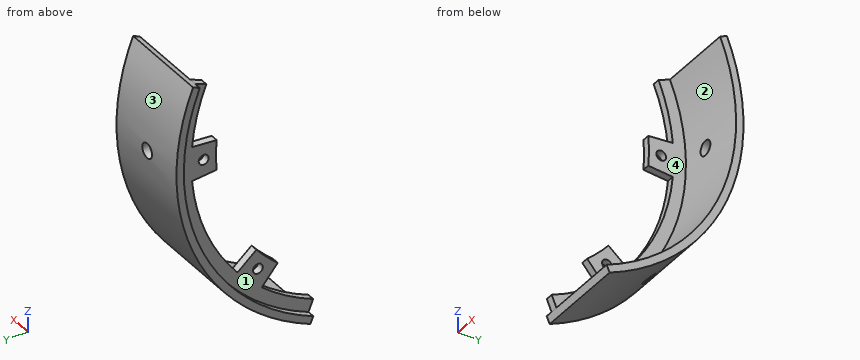
```python
from build123d import *

# Parameters (mm, degrees)
SKETCH5_R                = 2
BOSS_EXTRUDE2_DEPTH      = 3
BOSS_EXTRUDE3_DEPTH      = 30.8
BOSS_EXTRUDE3_DEPTH_BACK = 6
CUT_EXTRUDE1_START       = 84.947042212
CUT_EXTRUDE1_DEPTH       = 3.052957992
CIRPATTERN1_COUNT        = 8


# Read off the part's stored shape, not the designer's step: Cut-Extrude1
with BuildPart() as part:
    # Sketch5 → Boss-Extrude2 (new body)
    with BuildSketch(Plane(origin=(0, 0, 0), x_dir=(0, 0, -1), z_dir=(1, 0, 0))):
        with BuildLine():
            Line((-32.528091751, 78.529760263), (-30.614674589, 73.910362601))
            ThreePointArc((-30.614674589, 73.910362601), (-19.014871386, 77.707365585), (-6.97245942, 79.695575847))
            Line((-6.97245942, 79.695575847), (-6.100901992, 69.733628866))
            ThreePointArc((-6.100901992, 69.733628866), (0, 70), (6.100901992, 69.733628866))
            Line((6.100901992, 69.733628866), (6.97245942, 79.695575847))
            ThreePointArc((6.97245942, 79.695575847), (30.614674589, 73.910362601), (51.423008775, 61.28355545))
            Line((51.423008775, 61.28355545), (44.995132678, 53.623111018))
            ThreePointArc((44.995132678, 53.623111018), (49.497474683, 49.497474683), (53.623111018, 44.995132678))
            Line((53.623111018, 44.995132678), (61.28355545, 51.423008775))
            ThreePointArc((61.28355545, 51.423008775), (68.392949654, 41.501860653), (73.910362601, 30.614674589))
            Line((73.910362601, 30.614674589), (78.529760263, 32.528091751))
            ThreePointArc((78.529760263, 32.528091751), (32.528091751, 78.529760263), (-32.528091751, 78.529760263))
        make_face()
        with Locations((0, 75)):
            Circle(SKETCH5_R, mode=Mode.SUBTRACT)
        with Locations((53.033008589, 53.033008589)):
            Circle(SKETCH5_R, mode=Mode.SUBTRACT)
    extrude(amount=BOSS_EXTRUDE2_DEPTH)

    # Sketch6 → Boss-Extrude3 (add, two sides: drawn at the far end of the back side and taken through both)
    with BuildSketch(Plane(origin=(3, 0, 0), x_dir=(0, 0, -1), z_dir=(1, 0, 0)).offset(-BOSS_EXTRUDE3_DEPTH_BACK)):
        with BuildLine():
            Line((-33.776344001, 81.259821474), (-32.528091751, 78.529760263))
            ThreePointArc((-32.528091751, 78.529760263), (32.528091751, 78.529760263), (78.529760263, 32.528091751))
            Line((78.529760263, 32.528091751), (81.259821474, 33.776344001))
            ThreePointArc((81.259821474, 33.776344001), (33.575888915, 81.342852689), (-33.776344001, 81.259821474))
        make_face()
    extrude(amount=BOSS_EXTRUDE3_DEPTH + BOSS_EXTRUDE3_DEPTH_BACK)

    # Cut-Extrude1 outline → Cut-Extrude1 (cut)
    with BuildSketch(Plane(origin=(0, 0, 0), x_dir=(1, 0, 0), z_dir=(0, 1, 0)).offset(CUT_EXTRUDE1_START)):
        with BuildLine():
            add(Edge.make_bspline(
                [(15, 3), (14.207155752, 3), (13.431935871, 2.67467752), (12.32503645, 1.56757614), (12.000417509, 0.784253557), (11.999583343, -0.781056107), (12.317849893, -1.559926049), (13.437373681, -2.680577823), (14.215788964, -2.999721613), (15.78207965, -3.000278008), (16.565523239, -2.676042446), (17.673000882, -1.570710817), (17.999196633, -0.794471212), (18.000800287, 0.788392407), (17.676438527, 1.565317466), (16.569584029, 2.673938655), (15.792844248, 3), (15, 3)],
                knots=[0, 0, 0, 0, 0.125, 0.125, 0.25, 0.25, 0.375, 0.375, 0.5, 0.5, 0.625, 0.625, 0.75, 0.75, 0.875, 0.875, 1, 1, 1, 1], degree=3))
        make_face()
    cut_extrude1 = extrude(amount=CUT_EXTRUDE1_DEPTH, mode=Mode.SUBTRACT)

    # CirPattern1: Cut-Extrude1 ×8 about axis, 6 skipped
    cirpattern1_axis = Axis((0, 0, 0), (1, 0, 0))
    add([cut_extrude1.rotate(cirpattern1_axis, i * 360 / CIRPATTERN1_COUNT) for i in range(1, CIRPATTERN1_COUNT) if i not in (1, 2, 3, 4, 5, 6)], mode=Mode.SUBTRACT)


solid = part.part
```
Model file for the job. Use its own axes, mm. Face numbers are marked on the shaded views. A direction names the side the tool comes from. Coordinates: 2 decimals unless noted, no trailing zeros. Write each loop counter-clockwise with the first axis right and the second up, starting at its lowest first coordinate (ties: lowest second). Pieces come first, ordered by that corner, then holes. Notation, with made-up numbers: (44.25, 49) - (55.25, 49) arc R15 cw to (55.25, 66) - close; hole circle Ø4 at (-13.75, 7). An arc over 180 degrees is marked (long way). Use a Markdown table: item, result. Add a question column.
Item 1: Band-saw the part on B-B, the plane y = 47.5. Write the cut outline in (x, z).
Item 2: Drop flat-ended pins along their axis: pin 1 (12 mm diameter, centred on x = 3, z = -63.5, fed in from +Y); pin 2 (2.5 mm diameter, centred on y = 53.03, z = -53.03, fed in from -X); pin 3 (8 mm diameter, centred on x = 19, y = 52, fed in from +Z); pin 4 (5 mm diameter, centred on x = 4, z = -30, fed in from +Y). Give the stop position or say it passes through.
Item 3: Two-plate mould, pull along Z, no slides. Class the marked faces 3 and 4: pulls with the +Z half, pulls with the -Z half, needs draft (parallel to the pull), parting line crosses it, or undercut.
Item 4: 3-axis set-ups, long thin cutter, end or side, ignore diameter. For the marked faces 1 and 2: which of +Z, -Z, +X, -X, +Y, -Y reach the whole face in a straight line?
Item 5: Drill centre lines: line 1 along Y through (x, z) = (1.7, 0); line 2 along X through (y, z) = (51, -49.5); line 3 along Y through (x, z) = (21.5, -45). Where is each one in solid material? Low to high.
Item 6: Band-saw the part on C-C, the plane x = 10.5. Write the cut outline in (y, z), and give its area (3 significant figures).
Item 7: Band-saw the part on A-A, the plane z = 0. Give the number of separate pieces and of enclosed holes in the cut face, and give its area (3 significant figures).
Item 8: Band-saw the part on D-D, the plane y = 75. Write the cut outline in (x, z), and give its area (3 significant figures).
A:
| question | item | result |
|---|---|---|
| 1 | outline | (-3, -74.08) - (33.8, -74.08) - (33.8, -70.49) - (3, -70.49) - (3, -64.37) - (0, -64.37) - (0, -70.49) - (-3, -70.49) - close; (0, -56.61) - (3, -56.61) - (3, -51.42) - (0, -51.42) - close |
| 2 | pin 1 | stops at y = 66.62 |
| 2 | pin 2 | passes through |
| 2 | pin 3 | stops at z = -63.95 |
| 2 | pin 4 | stops at y = 83.59 |
| 3 | face 3 | parting line crosses it |
| 3 | face 4 | undercut |
| 4 | face 1 | -X, -Y |
| 4 | face 2 | +X, -Y |
| 5 | line 1 | y = 70 to 73, 77 to 88 |
| 5 | line 2 | x = 0 to 3 |
| 5 | line 3 | y = 72.11 to 75.62 |
| 6 | outline | (32.53, -78.53) - (33.78, -81.26) arc R88 ccw to (81.26, 33.78) - (78.53, 32.53) arc R85 cw to start |
| 6 | area | 408 mm² |
| 7 | separate pieces | 3 |
| 7 | enclosed holes | 0 |
| 7 | area | 125 mm² |
| 8 | outline | (-3, -46.03) - (33.8, -46.03) - (33.8, -40) - (3, -40) - (3, -27.84) - (0, -27.84) - (0, -40) - (-3, -40) - close; (0, -6.56) - (3, -6.56) - (3, -2) - (0, -2) - close; (0, 2) - (3, 2) - (3, 6.56) - (0, 6.56) - close; (0, 27.84) - (3, 27.84) - (3, 31.07) - (0, 31.07) - close |
| 8 | area | 296 mm² |
